Job drawing, mm, ordinate dimensions from the low corner. One solid piece. A direction names the side the tool comes from. Coordinates: 2 decimals unless noted, no trailing zeros. Loops run counter-clockwise (first coordinate to the right, second up) from the corner with the lowest first, then second, coordinate; pieces in that order, holes last. Notation, with made-up numbers: (55.25, 70.25) - (107.25, 70.25) arc R19 cw to (107.25, 100.25) - close; hole circle Ø1 at (73.25, 3.25). An arc over 180 degrees is marked (long way). Use a Markdown table: item, result. Add a question column.
1. Drop a flat-ended pin along its axis: pin 1 (2 mm diameter, centred on x = 40, z = 12.5, fed in from +Y). Give the stop position or say it passes through.
2. Band-saw the part on C-C, the plane x = 44. Give the cut face in (y, z), plus the area to 3 significant figures.
3. Band-saw the part on D-D, the plane x = 60. Give the cut face in (y, z).
4. Wall check: probe 1 along Z at (x, y) = (40, 18.2); probe 2 along Z at (x, y) = (60, 11.75); probe 3 along X at (y, z) = (7.5, 7.25). Give the ranges that are in metal, low to high. Write a range as [from, to].
5. Band-saw the part on A-A, the plane y = 11.75. Give the cut face in (x, z).
6. Pull direction Z, two halves, no side cores. Call the marked faces 3, 4, 5 and 6: pulls with the +Z half, pulls with the -Z half, needs draft (parallel to the pull), parting line crosses it, or undercut.
7. 3-axis set-ups, long thin cutter, end or side, ignore diameter. For the marked faces 1 and 2: which of +Z, -Z, +X, -X, +Y, -Y reach the whole face in a straight line?
8. Band-saw the part on B-B, the plane z = 9.5. Give the cut face in (x, y), plus the area to 3 significant figures.
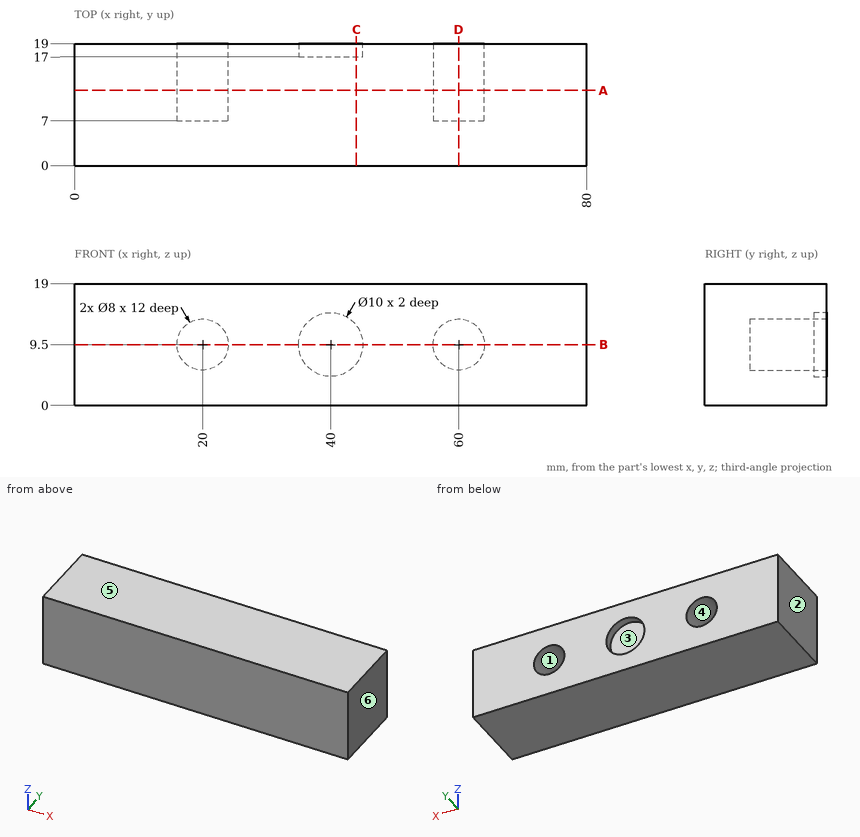
Geometry check:
| question | item | result |
|---|---|---|
| 1 | pin 1 | stops at y = 17 |
| 2 | outline | (0, 0) - (19, 0) - (19, 6.5) - (17, 6.5) - (17, 12.5) - (19, 12.5) - (19, 19) - (0, 19) - close |
| 2 | area | 349 mm^2 |
| 3 | outline | (0, 0) - (19, 0) - (19, 5.5) - (7, 5.5) - (7, 13.5) - (19, 13.5) - (19, 19) - (0, 19) - close |
| 4 | probe 1 | z = [0, 4.5], [14.5, 19] |
| 4 | probe 2 | z = [0, 5.5], [13.5, 19] |
| 4 | probe 3 | x = [0, 16.69], [23.31, 56.69], [63.31, 80] |
| 5 | outline | (0, 0) - (80, 0) - (80, 19) - (0, 19) - close; hole circle Ø8 at (20, 9.5); hole circle Ø8 at (60, 9.5) |
| 6 | face 3 | undercut |
| 6 | face 4 | undercut |
| 6 | face 5 | pulls with the +Z half |
| 6 | face 6 | needs draft |
| 7 | face 1 | +Y |
| 7 | face 2 | +Z, -Z, -X, +Y, -Y |
| 8 | outline | (0, 0) - (80, 0) - (80, 19) - (64, 19) - (64, 7) - (56, 7) - (56, 19) - (45, 19) - (45, 17) - (35, 17) - (35, 19) - (24, 19) - (24, 7) - (16, 7) - (16, 19) - (0, 19) - close |
| 8 | area | 1,310 mm^2 |
